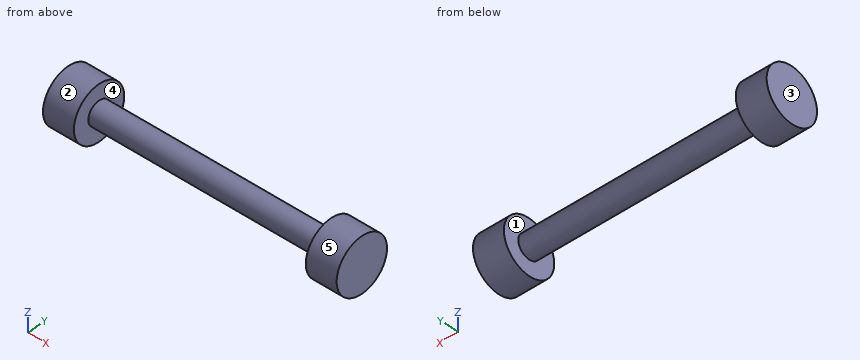
from build123d import *

# Parameters (mm, degrees)
F0_R     = 3.81
F1_DEPTH = 76.2
F3_R     = 8.89
F4_DEPTH = 10.16
F5_R     = 8.89
F6_DEPTH = 10.16


with BuildPart() as f1:
    # F0 (on Right) → F1 (new body)
    with BuildSketch(Plane.YZ):
        Circle(F0_R)
    extrude(amount=F1_DEPTH)

    # F3 (on face) → F4 (join)
    with BuildSketch(Plane(origin=(0, 0, 0), x_dir=(0, -1, 0), z_dir=(-1, 0, 0))):
        Circle(F3_R)
    extrude(amount=F4_DEPTH)

    # F5 (on face) → F6 (join)
    with BuildSketch(Plane.YZ.offset(76.2)):
        Circle(F5_R)
    extrude(amount=F6_DEPTH)


solid = f1.part
For this review, take the finished solid that the model builds, in its own axes (mm). Face numbers are marked on the shaded views. A direction names the side the tool comes from. Give positions to 0.01 mm unless a question says otherwise; leave off trailing zeros. Loops run counter-clockwise (first coordinate to the right, second up) from the corner with the lowest first, then second, coordinate; pieces in that order, holes last.
Item 1: Insertion check: pin 1 (8 mm diameter, centred on x = 35, z = 6.5, fed in from +Y); pin 2 (1 mm diameter, centred on x = 50, y = -6, fed in from +Z); pin 3 (5 mm diameter, centred on x = 45, z = 0, fed in from +Y); pin 4 (3 mm diameter, centred on x = 15, z = 0, fed in from -Y). Each pin has a flat end and moves straight along its axis. Give the tip position at first contact, or say it passes through.
Item 2: For line 1 along X through (y, z) = (-2.25, -7.25); line 2 along Z through (x, y) = (50.5, 0); line 3 along Y through (x, z) = (50, 2), list the stretches that pass through material, from the lowest coordinate up.
Item 3: Draft analysis for pull direction X (two halves, no side actions). For the marked faces 3, 4 and 5, state which applies: +X half, -X half, draft (parallel to the pull), parting line (faces both ways), or undercut.
Item 4: Take a section at D-D, the plane y = -5. State the section outline as (x, z) points.
Item 5: Take a section at C-C, the plane z = -5.25. State the section outline as (x, y) points, and give its area (3 significant figures).
Item 6: Take a section at A-A, the plane y = 0. State the section outline as (x, z) points.
Item 7: Tool access review of the marked faces 1 and 2: name each direction out of +Z, -Z, +X, -X, +Y, -Y from which nothing blocks a thin tool from reaching the whole face with its end or side.
Calculated:
1. pin 1: stops at y = 2.88
1. pin 2: passes through
1. pin 3: stops at y = 3.81
1. pin 4: stops at y = -3.81
2. line 1: x = -10.16 to 0, 76.2 to 86.36
2. line 2: z = -3.81 to 3.81
2. line 3: y = -3.24 to 3.24
3. face 3: -X half
3. face 4: undercut
3. face 5: draft
4. outline: (-10.16, -7.35) - (0, -7.35) - (0, 7.35) - (-10.16, 7.35) - close; (76.2, -7.35) - (86.36, -7.35) - (86.36, 7.35) - (76.2, 7.35) - close
5. outline: (-10.16, -7.17) - (0, -7.17) - (0, 7.17) - (-10.16, 7.17) - close; (76.2, -7.17) - (86.36, -7.17) - (86.36, 7.17) - (76.2, 7.17) - close
5. area: 292 mm2
6. outline: (-10.16, -8.89) - (0, -8.89) - (0, -3.81) - (76.2, -3.81) - (76.2, -8.89) - (86.36, -8.89) - (86.36, 8.89) - (76.2, 8.89) - (76.2, 3.81) - (0, 3.81) - (0, 8.89) - (-10.16, 8.89) - close
7. face 1: none
7. face 2: +X, -X
